Build history of the part. All positions in model axes, mm. Coordinates: 2 decimals unless noted, no trailing zeros. Order: outer loops, then holes, each group sorted by start corner. A loop starts at its lowest first (then second) coordinate and runs counter-clockwise, first axis right, second up. Notation, with made-up numbers: (87.5, 14.5) - (109.5, 14.5) arc R28 ccw to (109.5, 45.5) - close; hole circle Ø9 at (-22.75, -6). An arc over 180 degrees is marked (long way). Write each question's results on one line, items separated by ' | '. Start each with the question number.
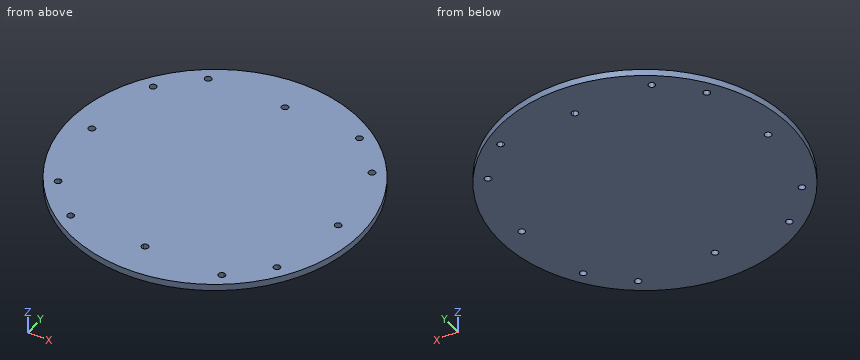
from build123d import *

# Parameters (mm, degrees)
F0_R     = 55
F0_R_2   = 1.25
F0_W     = 57.1
F0_H     = 57.1
F1_DEPTH = 2.5


with BuildPart() as f1:
    # F0 (on Top) → F1 (new body)
    with BuildSketch(Plane.XY):
        Circle(F0_R)
        with Locations((-46.5, 0)):
            Circle(F0_R_2, mode=Mode.SUBTRACT)
        with BuildLine():
            ThreePointArc((1, -41.3), (1.1858541226, -41.6547152925), (1.25, -42.05))
            ThreePointArc((1.25, -42.05), (-0.3952847075, -43.2358541226), (-1, -41.3))
            Line((-1, -41.3), (-27.3, -41.3))
            ThreePointArc((-27.3, -41.3), (-29.4338834765, -42.1838834765), (-28.55, -40.05))
            Line((-28.55, -40.05), (-28.55, -28.55))
            Line((-28.55, -28.55), (-40.05, -28.55))
            ThreePointArc((-40.05, -28.55), (-42.1838834765, -29.4338834765), (-41.3, -27.3))
            Line((-41.3, -27.3), (-41.3, 27.3))
            ThreePointArc((-41.3, 27.3), (-42.1838834765, 29.4338834765), (-40.05, 28.55))
            Line((-40.05, 28.55), (-28.55, 28.55))
            Line((-28.55, 28.55), (-28.55, 40.05))
            ThreePointArc((-28.55, 40.05), (-29.4338834765, 42.1838834765), (-27.3, 41.3))
            Line((-27.3, 41.3), (-1, 41.3))
            ThreePointArc((-1, 41.3), (-0.3952847075, 43.2358541226), (1.25, 42.05))
            ThreePointArc((1.25, 42.05), (1.1858541226, 41.6547152925), (1, 41.3))
            Line((1, 41.3), (27.3, 41.3))
            ThreePointArc((27.3, 41.3), (28.55, 42.55), (29.8, 41.3))
            ThreePointArc((29.8, 41.3), (29.4338834765, 40.4161165235), (28.55, 40.05))
            Line((28.55, 40.05), (28.55, 28.55))
            Line((28.55, 28.55), (40.05, 28.55))
            ThreePointArc((40.05, 28.55), (41.3, 29.8), (42.55, 28.55))
            ThreePointArc((42.55, 28.55), (42.1838834765, 27.6661165235), (41.3, 27.3))
            Line((41.3, 27.3), (41.3, -27.3))
            ThreePointArc((41.3, -27.3), (42.1838834765, -27.6661165235), (42.55, -28.55))
            ThreePointArc((42.55, -28.55), (41.3, -29.8), (40.05, -28.55))
            Line((40.05, -28.55), (28.55, -28.55))
            Line((28.55, -28.55), (28.55, -40.05))
            ThreePointArc((28.55, -40.05), (29.4338834765, -40.4161165235), (29.8, -41.3))
            ThreePointArc((29.8, -41.3), (28.55, -42.55), (27.3, -41.3))
            Line((27.3, -41.3), (1, -41.3))
        make_face(mode=Mode.SUBTRACT)
        with Locations((46.5, 0)):
            Circle(F0_R_2, mode=Mode.SUBTRACT)
        with BuildLine():
            Line((-28.55, 28.55), (28.55, 28.55))
            Line((28.55, 28.55), (28.55, 40.05))
            ThreePointArc((28.55, 40.05), (27.6661165235, 40.4161165235), (27.3, 41.3))
            Line((27.3, 41.3), (1, 41.3))
            ThreePointArc((1, 41.3), (0, 40.8), (-1, 41.3))
            Line((-1, 41.3), (-27.3, 41.3))
            ThreePointArc((-27.3, 41.3), (-27.6661165235, 40.4161165235), (-28.55, 40.05))
            Line((-28.55, 40.05), (-28.55, 28.55))
        make_face()
        Rectangle(F0_W, F0_H)
        with BuildLine():
            Line((-40.05, -28.55), (-28.55, -28.55))
            Line((-28.55, -28.55), (-28.55, 28.55))
            Line((-28.55, 28.55), (-40.05, 28.55))
            ThreePointArc((-40.05, 28.55), (-40.4161165235, 27.6661165235), (-41.3, 27.3))
            Line((-41.3, 27.3), (-41.3, -27.3))
            ThreePointArc((-41.3, -27.3), (-40.4161165235, -27.6661165235), (-40.05, -28.55))
        make_face()
        with BuildLine():
            ThreePointArc((-1, -41.3), (0, -40.8), (1, -41.3))
            Line((1, -41.3), (27.3, -41.3))
            ThreePointArc((27.3, -41.3), (27.6661165235, -40.4161165235), (28.55, -40.05))
            Line((28.55, -40.05), (28.55, -28.55))
            Line((28.55, -28.55), (-28.55, -28.55))
            Line((-28.55, -28.55), (-28.55, -40.05))
            ThreePointArc((-28.55, -40.05), (-27.6661165235, -40.4161165235), (-27.3, -41.3))
            Line((-27.3, -41.3), (-1, -41.3))
        make_face()
        with BuildLine():
            Line((28.55, 28.55), (28.55, -28.55))
            Line((28.55, -28.55), (40.05, -28.55))
            ThreePointArc((40.05, -28.55), (40.4161165235, -27.6661165235), (41.3, -27.3))
            Line((41.3, -27.3), (41.3, 27.3))
            ThreePointArc((41.3, 27.3), (40.4161165235, 27.6661165235), (40.05, 28.55))
            Line((40.05, 28.55), (28.55, 28.55))
        make_face()
    extrude(amount=F1_DEPTH)


solid = f1.part
Item 1: Probe probe 1 along X at (y, z) = (-42, 1.85); probe 2 along Y at (x, z) = (-41.3, 1.6); probe 3 along X at (y, z) = (28.55, 1.4). List the from-to ranges inside material, lowest first.
Item 2: Flat gauge pins, fed straight in: P1, Ø1, axis at y = -1, z = 0.5, coming from the +X side; P2, Ø1.5, axis at x = -28, z = 2, coming from the +Y side. Where does each tip first touch, or does it go through?
Item 3: Slice it at D-D (y = 34). Write the cut outline in (x, z), then the cut area to 3 significant figures.
Item 4: Slice it at B-B (z = 0.65). Count the separate pieces of the cut face and the enclosed holes in it, then the cut area to 3 significant figures.
Item 5: Slice it at A-A (y = 0). Write the cut outline in (x, z), then the cut area to 4 significant figures.
Item 6: Slice it at C-C (x = -46.5). Write the cut outline in (y, z), then the cut area to 3 significant figures.
Resolved:
1) probe 1: -35.51 to -29.59, -27.51 to -1.25, 1.25 to 27.51, 29.59 to 35.51 | probe 2: -36.32 to -29.8, -27.3 to 27.3, 29.8 to 36.32 | probe 3: -47.01 to -42.55, -40.05 to 40.05, 42.55 to 47.01
2) P1: x = 55 | P2: y = 47.77
3) outline: (-43.23, 0) - (43.23, 0) - (43.23, 2.5) - (-43.23, 2.5) - close | area: 216 mm^2
4) separate pieces: 1 | enclosed holes: 12 | area: 9,440 mm^2
5) outline: (-55, 0) - (-47.75, 0) - (-47.75, 2.5) - (-55, 2.5) - close; (-45.25, 0) - (45.25, 0) - (45.25, 2.5) - (-45.25, 2.5) - close; (47.75, 0) - (55, 0) - (55, 2.5) - (47.75, 2.5) - close | area: 262.5 mm^2
6) outline: (-29.37, 0) - (-1.25, 0) - (-1.25, 2.5) - (-29.37, 2.5) - close; (1.25, 0) - (29.37, 0) - (29.37, 2.5) - (1.25, 2.5) - close | area: 141 mm^2
